Design review of the part built by this model. Coordinates are the model's own, in mm. A direction names the side the tool comes from. Coordinates: 2 decimals unless noted, no trailing zeros. Loops run counter-clockwise (first coordinate to the right, second up) from the corner with the lowest first, then second, coordinate; pieces in that order, holes last. Notation, with made-up numbers: M -19.5,34 L 14.5,34 A15 cw 14.5,47 Z; hole C 71,14.5 d5. An arc over 180 degrees is marked long. Answer as a JSON object with one key per item and string values. Group by question number.
1. Consider section A-A (z = 0). State the section outline as (x, y) points.
2. Machinability: for faces 4 (the flat face through (3, -6.5, -4)), 5 (the cylindrical face through (-5.894, -4.528, 0.259)), 6 (the flat face through (4.3, 2.5, -4.3)), which of the approach directions +Z, -Z, +X, -X, +Y, -Y give a long, thin tool a straight path to every point of the face, cutting with its end or side? Answer none if there is none.
3. To check wall thickness, follow probe 1 along Z at (x, y) = (0, 1.75); probe 2 along Y at (x, z) = (-3, 9); probe 3 along Z at (x, y) = (0.25, -6). State the ranges of each line that lie inside material, in increasing order.
4. Insertion check: pin 1 (2 mm diameter, centred on x = 8, y = 4.5, fed in from -Z); pin 2 (2 mm diameter, centred on x = -2.5, z = 7.5, fed in from -Y); pin 3 (8 mm diameter, centred on x = -5.5, z = 4, fed in from +Y); pin 4 (2 mm diameter, centred on y = 2.5, z = 3.5, fed in from +X). Each pin has a flat end and moves straight along its axis. Give the tip position at first contact, or say it passes through.
5. Consider section C-C (y = -5.5). State the section outline as (x, z) points, then the cut area to 3 significant figures.
6. Draft analysis for pull direction Z (two halves, no side actions). For faces 1 (the cylindrical face through (-5.894, 4.127, 0.259)), 2 (the flat face through (-2, 6.5, -4)), 3 (the cylindrical face through (2.285, 0.091, 3.584)), state which applies: +Z half, -Z half, draft (parallel to the pull), parting line (faces both ways), or undercut.
7. Consider section D-D (x = -8). State the section outline as (y, z) points.
8. Consider section B-B (x = 0). State the section outline as (y, z) points.
from build123d import *

# Parameters (mm, degrees)
F0_R     = 10
F0_R_2   = 5.9
F1_DEPTH = 2.5
F0_R_3   = 4.25
F2_DEPTH = 6.5
F3_R     = 0.7


with BuildPart() as f1:
    # F0 (on Front) → F1 (new body, symmetric)
    with BuildSketch(Plane.XZ):
        Circle(F0_R)
        Circle(F0_R_2, mode=Mode.SUBTRACT)
    extrude(amount=F1_DEPTH, both=True)

    # F0 (on Front) → F2 (join, symmetric)
    with BuildSketch(Plane.XZ):
        Circle(F0_R_2)
        Circle(F0_R_3, mode=Mode.SUBTRACT)
    extrude(amount=F2_DEPTH, both=True)

    # F3
    f3_edges = [f1.edges().sort_by_distance(p)[0] for p in [
        (-5.9, 6.5, 0),
    ]]
    fillet(f3_edges, radius=F3_R)


solid = f1.part
Findings below:
{
 "1": {"outline": "M -10,-2.5 L -5.9,-2.5 L -5.9,-6.5 L -4.25,-6.5 L -4.25,6.5 L -5.2,6.5 A0.7 ccw -5.9,5.8 L -5.9,2.5 L -10,2.5 Z; M 4.25,-6.5 L 5.9,-6.5 L 5.9,-2.5 L 10,-2.5 L 10,2.5 L 5.9,2.5 L 5.9,5.8 A0.7 ccw 5.2,6.5 L 4.25,6.5 Z"},
 "2": {"face 4": "+Z, -Z, +X, -X, -Y", "face 5": "-Y", "face 6": "+Y"},
 "3": {"probe 1": "z = -10 to -4.25, 4.25 to 10", "probe 2": "y = -2.5 to 2.5", "probe 3": "z = -5.89 to -4.24, 4.24 to 5.89"},
 "4": {"pin 1": "passes through", "pin 2": "stops at y = -2.5", "pin 3": "stops at y = 6.5", "pin 4": "stops at x = 9.68"},
 "5": {"outline": "C 0,0 d11.8; hole C 0,0 d8.5", "area": "52.6 mm^2"},
 "6": {"face 1": "parting line", "face 2": "draft", "face 3": "undercut"},
 "7": {"outline": "M -2.5,-6 L 2.5,-6 L 2.5,6 L -2.5,6 Z"},
 "8": {"outline": "M -6.5,-5.9 L -2.5,-5.9 L -2.5,-10 L 2.5,-10 L 2.5,-5.9 L 5.8,-5.9 A0.7 ccw 6.5,-5.2 L 6.5,-4.25 L -6.5,-4.25 Z; M -6.5,4.25 L 6.5,4.25 L 6.5,5.2 A0.7 ccw 5.8,5.9 L 2.5,5.9 L 2.5,10 L -2.5,10 L -2.5,5.9 L -6.5,5.9 Z"}
}
